Here's how the part is built. I have some questions about the finished solid (model axes, mm). A direction names the side the tool comes from. Give positions to 0.01 mm unless a question says otherwise; leave off trailing zeros. Write each loop counter-clockwise with the first axis right and the second up, starting at its lowest first coordinate (ties: lowest second). Pieces come first, ordered by that corner, then holes. Notation, with made-up numbers: (54.25, 13.5) -> (69.25, 13.5) arc R18 ccw to (69.25, 46.5) -> close; hole circle Ø9 at (6, -13.5). An arc over 180 degrees is marked (long way). Return JSON: item names as keys, results as strings.
Autodesk Inventor part; units mm, degrees
ref_plane "ROD_BA_XY" through (10, 0, 0) normal (-1, 0, 0) x (0, 0, -1)
ref_plane "ROD_BA_YZ" through (10, 0, 0) normal (0, 0, -1) x (0, -1, 0)
ref_plane "ROD_BA_ZX" through (10, 0, 0) normal (0, -1, 0) x (-1, 0, 0)
sketch "Sketch_5" plane through (0, 0, 0) normal (0, 0, 1) x (1, 0, 0)
  line L0 (60.5, 0) -> (0, 0)
  line L1 (0, 0) -> (0, 2.0095)
  line L2 (0, 2.0095) -> (0.4905, 2.5)
  line L3 (0.4905, 2.5) -> (15, 2.5)
  line L4 (15, 2.5) -> (15, 2.067)
  line L5 (15, 2.067) -> (16.5, 2.067)
  line L6 (16.5, 2.067) -> (16.5, 2.5)
  line L7 (16.5, 2.5) -> (55.5, 2.5)
  line L8 (55.5, 2.5) -> (55.5, 8)
  line L9 (55.5, 8) -> (60.5, 8)
  line L10 (60.5, 8) -> (60.5, 0)
  line L11 (60.5, 0) -> (0, 0)
revolve "Revolution1" add sketch "Sketch_5" angle 360 about axis through (60.5, 0, 0) along (1, 0, 0)
thread "Thread1"
ref_plane "ROD_BA_XY" through (10, 0, 0) normal (-1, 0, 0) x (0, 0, -1)
ref_plane "ROD_BA_YZ" through (10, 0, 0) normal (0, 0, -1) x (0, -1, 0)
ref_plane "ROD_BA_ZX" through (10, 0, 0) normal (0, -1, 0) x (-1, 0, 0)
ref_plane "ROD_BODY_XY" through (28, 0, 0) normal (1, 0, 0) x (0, 0, -1)
ref_plane "ROD_BODY_YZ" through (28, 0, 0) normal (0, 0, -1) x (0, 1, 0)
ref_plane "ROD_BODY_ZX" through (28, 0, 0) normal (0, 1, 0) x (1, 0, 0)
ref_plane "rodnt1_XY" through (7.5, 0, 0) normal (1, 0, 0) x (0, 0, -1)
ref_plane "rodnt1_YZ" through (7.5, 0, 0) normal (0, 0, -1) x (0, 1, 0)
ref_plane "rodnt1_ZX" through (7.5, 0, 0) normal (0, 1, 0) x (1, 0, 0)
properties part number "CJ2B16-15Z_ROD"
1. For pin 1 Ø2 at (x, y) = (16, -0.5) entering from -Z; pin 2 Ø8 at (x, z) = (38.5, -3) entering from -Y; pin 3 Ø2.5 at (y, z) = (-1, 0) entering from -X; pin 4 Ø8 at (x, y) = (37.5, -1) entering from +Z, each with a flat end and sliding along its axis, tell me the tip position at first contact or that it passes through.
Taken from the geometry:
{"pin 1": "stops at z = -2.5", "pin 2": "stops at y = -2.5", "pin 3": "stops at x = 0", "pin 4": "stops at z = 2.5"}
2. Suppose I cut it at A-A, the plane y = 0. List the corners of the cut face in (x, z) for me.
Taken from the geometry:
{"outline": "(0, -2.01) -> (0.49, -2.5) -> (15, -2.5) -> (15, -2.07) -> (16.5, -2.07) -> (16.5, -2.5) -> (55.5, -2.5) -> (55.5, -8) -> (60.5, -8) -> (60.5, 8) -> (55.5, 8) -> (55.5, 2.5) -> (16.5, 2.5) -> (16.5, 2.07) -> (15, 2.07) -> (15, 2.5) -> (0.49, 2.5) -> (0, 2.01) -> close"}
3. Suppose I cut it at D-D, the plane y = -3.75. List the corners of the cut face in (x, z) for me.
Taken from the geometry:
{"outline": "(55.5, -7.07) -> (60.5, -7.07) -> (60.5, 7.07) -> (55.5, 7.07) -> close"}
4. Which directions (+Z, -Z, +X, -X, +Y, -Y) give clear straight access to the entire face, cutting with the end or side of a thin tool? Please do faces 4 (the face through (7.85, -0.54, -2.44)), 5 (the face through (60.5, 0, 0)), 6 (the face through (16.5, -1, 2)).
Taken from the geometry:
{"face 4": "-X", "face 5": "+Z, -Z, +X, +Y, -Y", "face 6": "none"}
5. Suppose I cut it at C-C, the plane x = 7. List the corners of the cut face in (y, z) for me.
Taken from the geometry:
{"outline": "circle Ø5 at (0, 0)"}
6. If I drill on line 1 (Z direction, x = 18.5, y = 0); line 2 (Y direction, x = 49, z = 1.5); line 3 (X direction, y = -1.5, z = -2.25), over which ranges is the centre line in solid material (lowest first)? Write a range as [from, to].
Taken from the geometry:
{"line 1": "z = [-2.5, 2.5]", "line 2": "y = [-2, 2]", "line 3": "x = [55.5, 60.5]"}
7. If we mould it in two halves opening along X, with no side actions, what happens to faces 1 (the face through (0, 0, 0)), 2 (the face through (15.76, -1.64, -1.26)), 3 (the face through (36.27, -0.54, -2.44))? For each: released by +X, released by -X, zero draft, split by the parting line, or undercut.
Taken from the geometry:
{"face 1": "released by -X", "face 2": "undercut", "face 3": "zero draft"}
